from build123d import *

# Parameters (mm, degrees)
F1_DEPTH = 914.4
F3_DEPTH = 38.101


with BuildPart() as f1:
    # F0 (on Front) → F1 (new body)
    with BuildSketch(Plane.XZ):
        Polygon((0, 38.1), (0, 0), (38.1, 0), (38.1, 4.7625), (4.7625, 4.7625), (4.7625, 38.1), align=None)
    extrude(amount=-F1_DEPTH)

    # F2 (on face) → F3 (cut, through all)
    with BuildSketch(Plane(origin=(0, 0, 0), x_dir=(0, -1, 0), z_dir=(-1, 0, 0))):
        Polygon((0, 38.1), (-38.1, 38.1), (0, 0), align=None)
        Polygon((-876.3, 38.1), (-914.4, 38.1), (-914.4, 0), align=None)
    extrude(amount=-F3_DEPTH, mode=Mode.SUBTRACT)


solid = f1.part
Here's how the part is built. I have some questions about the finished solid (model axes, mm). A direction names the side the tool comes from. Round coordinates to 2 decimals unless told otherwise and drop trailing zeros. Write each loop counter-clockwise with the first axis right and the second up, starting at its lowest first coordinate (ties: lowest second). Pieces come first, ordered by that corner, then holes.
1. Suppose I cut it at C-C (x = 12.5). List the corners of the cut face in (y, z) for me, and give its area (3 significant figures).
2. Will these pins go through, and if not, where does the flat tip stop? pin 1 Ø1.5 at (x, y) = (12.5, 365) entering from +Z; pin 2 Ø12 at (y, z) = (362.5, 30.5) entering from +X.
3. Suppose I cut it at A-A (y = 526.5). List the corners of the cut face in (x, z) for me, and give its area (3 significant figures).
4. For faces 1 (the flat face through (3.4, 903.9, 10.5)), 2 (the flat face through (4.762, 451, 21)), which set-ups out of +Z, -Z, +X, -X, +Y, -Y let a thin tool reach every point of the face, with its end or its side?
5. I need wall thicknesses on L1, parallel to X at y = 291, z = 25.5. Which ranges of the line are inside material? Lowest first, please.
6. Suppose I cut it at B-B (z = 24). List the corners of the cut face in (x, y) for me, and give its area (3 significant figures).
Answer sheet:
1. outline: (0, 0) - (914.4, 0) - (909.64, 4.76) - (4.76, 4.76) - close
1. area: 4,330 mm2
2. pin 1: stops at z = 4.76
2. pin 2: stops at x = 4.76
3. outline: (0, 0) - (38.1, 0) - (38.1, 4.76) - (4.76, 4.76) - (4.76, 38.1) - (0, 38.1) - close
3. area: 340 mm2
4. face 1: +Z, +X, -X, +Y
4. face 2: +Z, +X, +Y, -Y
5. L1: x = 0 to 4.76
6. outline: (0, 24) - (4.76, 24) - (4.76, 890.4) - (0, 890.4) - close
6. area: 4,130 mm2
